Input: part model. Units: mm. Frame: model coordinates. A direction names the side the tool comes from. Give positions to 0.01 mm unless a question says otherwise; leave off trailing zeros. Write each loop counter-clockwise with the first axis right and the second up, starting at its lowest first coordinate (ties: lowest second). Pieces come first, ordered by that corner, then holes. Notation, with made-up numbers: (26.5, -33.5) - (67.5, -33.5) arc R13 cw to (67.5, -13.5) - close; hole circle Ø8 at (61.25, 50.5). An arc over 180 degrees is marked (long way). Use a Markdown table: item, result. Add a question column.
1. Section query B-B, the plane y = -10.5. Return loops of the section in (x, z).
2. Section query D-D, the plane z = 62. Return loops of the section in (x, y).
3. Section query C-C, the plane y = 7. Return loops of the section in (x, z).
4. Material intervals for probe 1 along Y at (x, z) = (7.9, 50.5); probe 2 along X at (y, z) = (-10.5, 50.35); probe 3 along Z at (x, y) = (13, 17.5), sorted ascending.
5. Set-up query: faces 1 (the flat face through (2, 5, 48.5)), 2 (the flat face through (2, 7, 46.5)), 3 (the flat face through (22, 14.25, 58)). Return all of +Z, -Z, +X, -X, +Y, -Y with unobstructed straight access to the full face (end or side cutting, diameter ignored); none if empty.
6. Section query A-A, the plane x = 7.9. Return loops of the section in (y, z), plus the area to 3 significant figures.
7. Mould query, pull axis Y, two halves, no side actions, for faces 4 (the flat face through (22, -0.25, 58)), 5 (the cylindrical face through (7.466, 22.548, 50.406)), 6 (the cylindrical face through (-6.086, 7.616, 59.633)), 7 (the flat face through (0, 7, 40)). Classes: released by +Y, released by -Y, zero draft, split by the parting line, or undercut.
8. Pin query (flat end, axial travel): pin 1 (2 mm diameter, centred on y = 7.5, z = 48.5, fed in from -X); pin 2 (0.6 mm diameter, centred on x = 2, y = 7, fed in from -Z); pin 3 (8 mm diameter, centred on x = 12, y = 8.5, fed in from -Z); pin 4 (3.5 mm diameter, centred on x = 7.9, y = -10.5, fed in from +Z). Return the tip coordinate at first contact, or that it passes through.
```python
from build123d import *

# Parameters (mm, degrees)
CYLINDER017_R     = 2
CYLINDER017_DEPTH = 20
CYLINDER016_R     = 2
CYLINDER016_DEPTH = 20
CYLINDER019_R     = 4.5
CYLINDER019_DEPTH = 19.5
BOX013_W          = 7
BOX013_H          = 42
BOX013_DEPTH      = 0.8
FILLET012_R       = 3
FILLET013_R       = 3
FILLET014_R       = 3
FILLET015_R       = 3
BOX012_W          = 10
BOX012_H          = 14.5
BOX012_DEPTH      = 16.5
CYLINDER015_R     = 14
CYLINDER015_DEPTH = 19
BOX014_W          = 10
BOX014_H          = 10
BOX014_DEPTH      = 10
BOX015_W          = 10
BOX015_H          = 10
BOX015_DEPTH      = 10
CYLINDER018_R     = 2.7
CYLINDER018_DEPTH = 28


with BuildPart() as cylinder017:
    # Cylinder017 → Cylinder017 (new body)
    with BuildSketch(Plane(origin=(0, -17.5, 14), x_dir=(1, 0, 0), z_dir=(0, 0, 1))):
        Circle(CYLINDER017_R)
    extrude(amount=CYLINDER017_DEPTH)


with BuildPart() as cylinder016:
    # Cylinder016 → Cylinder016 (new body)
    with BuildSketch(Plane(origin=(0, 17.5, 14), x_dir=(1, 0, 0), z_dir=(0, 0, 1))):
        Circle(CYLINDER016_R)
    extrude(amount=CYLINDER016_DEPTH)


with BuildPart() as shaft_boss003:
    # Cylinder019 → Cylinder019 (new body)
    with BuildSketch(Plane(origin=(-8, 0, 1), x_dir=(1, 0, 0), z_dir=(0, 0, 1))):
        Circle(CYLINDER019_R)
    extrude(amount=CYLINDER019_DEPTH)


with BuildPart() as fillet015:
    # Box013 → Box013 (new body)
    with BuildSketch(Plane(origin=(-3.5, -21, 18.2), x_dir=(1, 0, 0), z_dir=(0, 0, 1))):
        with Locations((3.5, 21)):
            Rectangle(BOX013_W, BOX013_H)
    extrude(amount=BOX013_DEPTH)

    # Fillet012
    fillet012_edges = [fillet015.edges().sort_by_distance(p)[0] for p in [
        (3.5, -21, 18.6),
    ]]
    fillet(fillet012_edges, radius=FILLET012_R)

    # Fillet013
    fillet013_edges = [fillet015.edges().sort_by_distance(p)[0] for p in [
        (-3.5, -21, 18.6),
    ]]
    fillet(fillet013_edges, radius=FILLET013_R)

    # Fillet014
    fillet014_edges = [fillet015.edges().sort_by_distance(p)[0] for p in [
        (-3.5, 21, 18.6),
    ]]
    fillet(fillet014_edges, radius=FILLET014_R)

    # Fillet015
    fillet015_edges = [fillet015.edges().sort_by_distance(p)[0] for p in [
        (3.5, 21, 18.6),
    ]]
    fillet(fillet015_edges, radius=FILLET015_R)


with BuildPart() as cube012:
    # Box012 → Box012 (new body)
    with BuildSketch(Plane(origin=(5.5, -7.25, 2.5), x_dir=(1, 0, 0), z_dir=(0, 0, 1))):
        with Locations((5, 7.25)):
            Rectangle(BOX012_W, BOX012_H)
    extrude(amount=BOX012_DEPTH)


with BuildPart() as motor_body003:
    # Cylinder015 → Cylinder015 (new body)
    with BuildSketch(Plane.XY):
        Circle(CYLINDER015_R)
    extrude(amount=CYLINDER015_DEPTH)

    # Fusion012: union Cube012
    add(cube012.part)

    # Fusion013: union Fillet015
    add(fillet015.part)

    # Fusion014: union shaft-boss003
    add(shaft_boss003.part)

    # Cut014: cut Cylinder016
    add(cylinder016.part, mode=Mode.SUBTRACT)

    # Cut015: cut Cylinder017
    add(cylinder017.part, mode=Mode.SUBTRACT)


with BuildPart() as cube014:
    # Box014 → Box014 (new body)
    with BuildSketch(Plane(origin=(-6.4, -5, 22.5), x_dir=(1, 0, 0), z_dir=(0, 0, 1))):
        with Locations((5, 5)):
            Rectangle(BOX014_W, BOX014_H)
    extrude(amount=BOX014_DEPTH)


with BuildPart() as cube015:
    # Box015 → Box015 (new body)
    with BuildSketch(Plane(origin=(-19.6, -5, 22.5), x_dir=(1, 0, 0), z_dir=(0, 0, 1))):
        with Locations((5, 5)):
            Rectangle(BOX015_W, BOX015_H)
    extrude(amount=BOX015_DEPTH)


with BuildPart() as obj1:
    # Cylinder018 → Cylinder018 (new body)
    with BuildSketch(Plane(origin=(-8, 0, 1), x_dir=(1, 0, 0), z_dir=(0, 0, 1))):
        Circle(CYLINDER018_R)
    extrude(amount=CYLINDER018_DEPTH)

    # Cut012: cut Cube015
    add(cube015.part, mode=Mode.SUBTRACT)

    # Cut013: cut Cube014
    add(cube014.part, mode=Mode.SUBTRACT)

    # Fusion015: union motor-body003
    add(motor_body003.part)


with BuildPart() as obj1_1:
    # Fusion015 placement: moved
    add(obj1.part.moved(Location((7.9, 7, 7))))


with BuildPart() as obj2:
    # Part__Mirroring: instance of obj1
    add(obj1_1.part.mirror(Plane(origin=(0, 0, 0), x_dir=(0, 1, 0), z_dir=(0, 0, 1))))


with BuildPart() as obj2_1:
    # Part__Mirroring placement: moved
    add(obj2.part.moved(Location((0, 0, 76))))


solid = obj2_1.part
```
Result sheet:
| question | item | result |
|---|---|---|
| 1 | outline | (4.4, 50) - (5.9, 50) - (5.9, 50.8) - (4.4, 50.8) - close; (9.9, 50) - (11.4, 50) - (11.4, 50.8) - (9.9, 50.8) - close |
| 2 | outline | (19.88, -0.25) - (23.4, -0.25) - (23.4, 14.25) - (19.88, 14.25) arc R14 ccw (long way) to start |
| 3 | outline | (-6.1, 50) - (-4.6, 50) - (-4.6, 48.5) - (-2.8, 48.5) - (-2.8, 46.5) - (-1.7, 46.5) - (-1.7, 40) - (1.5, 40) - (1.5, 46.5) - (2.6, 46.5) - (2.6, 48.5) - (4.4, 48.5) - (4.4, 50) - (23.4, 50) - (23.4, 66.5) - (21.9, 66.5) - (21.9, 69) - (-6.1, 69) - close |
| 4 | probe 1 | y = -14 to -12.5, -8.5 to 22.5, 26.5 to 28 |
| 4 | probe 2 | x = 4.4 to 5.9, 9.9 to 11.4 |
| 4 | probe 3 | z = 50 to 69 |
| 5 | face 1 | -Z |
| 5 | face 2 | -Z, +X, +Y, -Y |
| 5 | face 3 | +Z, -Z, +X, +Y |
| 6 | outline | (-14, 50) - (-12.5, 50) - (-12.5, 50.8) - (-14, 50.8) - close; (-8.5, 50) - (22.5, 50) - (22.5, 50.8) - (21, 50.8) - (21, 69) - (-7, 69) - (-7, 50.8) - (-8.5, 50.8) - close; (26.5, 50) - (28, 50) - (28, 50.8) - (26.5, 50.8) - close |
| 6 | area | 537 mm² |
| 7 | face 4 | released by -Y |
| 7 | face 5 | undercut |
| 7 | face 6 | split by the parting line |
| 7 | face 7 | zero draft |
| 8 | pin 1 | stops at x = -4.6 |
| 8 | pin 2 | stops at z = 46.5 |
| 8 | pin 3 | stops at z = 50 |
| 8 | pin 4 | passes through |
